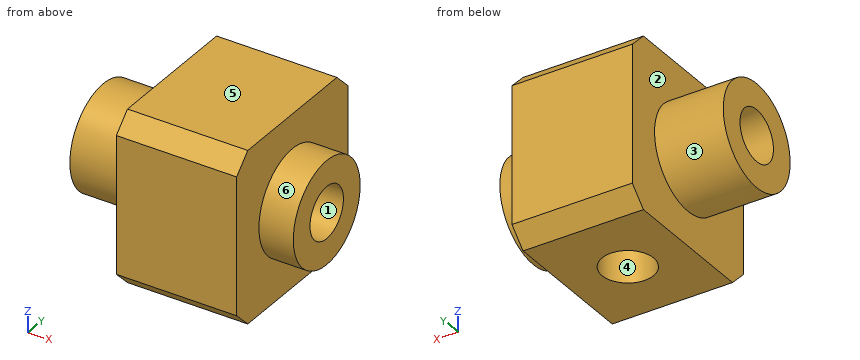
from build123d import *

# Parameters (mm, degrees)
SKETCH1_W           = 10
SKETCH1_H           = 10
BOSS_EXTRUDE1_DEPTH = 13
SKETCH2_R           = 15.353568197
SKETCH2_R_2         = 3
CUT_EXTRUDE1_DEPTH  = 2
CUT_EXTRUDE2_START  = -4
SKETCH3_R           = 15.635411304
SKETCH3_R_2         = 3
CUT_EXTRUDE2_DEPTH  = 4
SKETCH4_R           = 1.5
CUT_EXTRUDE3_DEPTH  = 15.798648587
CHAMFER1_SIZE       = 1
CUT_EXTRUDE4_START  = 5
SKETCH5_R           = 1.5
CUT_EXTRUDE4_DEPTH  = 2


with BuildPart() as part:
    # Sketch1 → Boss-Extrude1 (new body)
    with BuildSketch(Plane(origin=(0, 0, 0), x_dir=(0, 0, -1), z_dir=(1, 0, 0))):
        Rectangle(SKETCH1_W, SKETCH1_H)
    extrude(amount=-BOSS_EXTRUDE1_DEPTH)

    # Sketch2 → Cut-Extrude1 (cut)
    with BuildSketch(Plane(origin=(0, 0, 0), x_dir=(0, 0, -1), z_dir=(1, 0, 0))):
        Circle(SKETCH2_R)
        Circle(SKETCH2_R_2, mode=Mode.SUBTRACT)
    extrude(amount=-CUT_EXTRUDE1_DEPTH, mode=Mode.SUBTRACT)

    # Sketch3 → Cut-Extrude2 (cut)
    with BuildSketch(Plane.ZY.offset(13).offset(CUT_EXTRUDE2_START)):
        Circle(SKETCH3_R)
        with Locations(Location((0, 0, 0), (0, 0, 180))):
            Circle(SKETCH3_R_2, mode=Mode.SUBTRACT)
    extrude(amount=CUT_EXTRUDE2_DEPTH, mode=Mode.SUBTRACT)

    # Sketch4 → Cut-Extrude3 (cut, through all)
    with BuildSketch(Plane(origin=(0, 0, 0), x_dir=(0, 0, -1), z_dir=(1, 0, 0))):
        Circle(SKETCH4_R)
    extrude(amount=-CUT_EXTRUDE3_DEPTH, mode=Mode.SUBTRACT)

    # Chamfer1
    chamfer1_edges = [part.edges().sort_by_distance(p)[0] for p in [
        (-5.5, -5, -5),
        (-5.5, -5, 5),
        (-5.5, 5, -5),
        (-5.5, 5, 5),
    ]]
    chamfer(chamfer1_edges, length=CHAMFER1_SIZE)

    # Sketch5 → Cut-Extrude4 (cut)
    with BuildSketch(Plane(origin=(0, 0, 0), x_dir=(-1, 0, 0), z_dir=(0, 0, -1)).offset(CUT_EXTRUDE4_START)):
        with Locations((5.5, 0)):
            Circle(SKETCH5_R)
    extrude(amount=-CUT_EXTRUDE4_DEPTH, mode=Mode.SUBTRACT)


solid = part.part
The listing builds one solid part. Answer for the finished solid, in the listing's coordinates (mm). Face numbers are marked on the shaded views. A direction names the side the tool comes from. Give positions to 0.01 mm unless a question says otherwise; leave off trailing zeros. Write each loop counter-clockwise with the first axis right and the second up, starting at its lowest first coordinate (ties: lowest second). Pieces come first, ordered by that corner, then holes.
Item 1: Find the intervals of material crossed by line 1 along Y through (x, z) = (-5.5, 0); line 2 along X through (y, z) = (-3.75, 3.5); line 3 along Z through (x, y) = (-5, -1.25), in increasing order.
Item 2: Section D-D, the plane z = -3.25 is taken. Write down the section's boundary in (x, y), plus the area to 3 significant figures.
Item 3: Section A-A, the plane z = 0 is taken. Write down the section's boundary in (x, y).
Item 4: Section C-C, the plane x = -5.5 is taken. Write down the section's boundary in (y, z).
Item 5: Determine the mould class of the marked faces 1, 2 and 3 for opening direction Y: released by +Y, released by -Y, zero draft, split by the parting line, or undercut.
Item 6: Which of the six approach directions +Z, -Z, +X, -X, +Y, -Y give full straight-line access (tool end or side, diameter ignored) to the marked faces 4, 5 and 6?
Item 7: Section B-B, the plane y = 0 is taken. Write down the section's boundary in (x, z), plus the area to 3 significant figures.
Completed:
1. line 1: y = -5 to -1.5, 1.5 to 5
1. line 2: x = -9 to -2
1. line 3: z = -3 to -0.83, 0.83 to 5
2. outline: (-9, -5) - (-2, -5) - (-2, 5) - (-9, 5) - close; hole circle Ø3 at (-5.5, 0)
2. area: 62.9 mm2
3. outline: (-13, -3) - (-9, -3) - (-9, -5) - (-2, -5) - (-2, -3) - (0, -3) - (0, -1.5) - (-13, -1.5) - close; (-13, 1.5) - (0, 1.5) - (0, 3) - (-2, 3) - (-2, 5) - (-9, 5) - (-9, 3) - (-13, 3) - close
4. outline: (-5, -4) - (-4, -5) - (-1.5, -5) - (-1.5, -3) - (1.5, -3) - (1.5, -5) - (4, -5) - (5, -4) - (5, 4) - (4, 5) - (-4, 5) - (-5, 4) - close; hole circle Ø3 at (0, 0)
5. face 1: undercut
5. face 2: zero draft
5. face 3: split by the parting line
6. face 4: -Z
6. face 5: +Z, +X, -X, +Y, -Y
6. face 6: +X
7. outline: (-13, -3) - (-9, -3) - (-9, -5) - (-7, -5) - (-7, -3) - (-4, -3) - (-4, -5) - (-2, -5) - (-2, -3) - (0, -3) - (0, -1.5) - (-13, -1.5) - close; (-13, 1.5) - (0, 1.5) - (0, 3) - (-2, 3) - (-2, 5) - (-9, 5) - (-9, 3) - (-13, 3) - close
7. area: 61.0 mm2
